Can you work these out from the model? Positions are in its coordinate system, mm. A direction names the side the tool comes from. Round coordinates to 2 decimals unless told otherwise and drop trailing zeros. Loops run counter-clockwise (first coordinate to the right, second up) from the corner with the lowest first, then second, coordinate; pieces in that order, holes last. Notation, with made-up numbers: M 28,1 L 35,1 A12 cw 35,11 Z; hole C 20.25,73 d9. An arc over 180 degrees is marked long. Use a Markdown table: item, result. Add a question column.
```python
from build123d import *

# Parameters (mm, degrees)
SKETCH2_W               = 1.4224
SKETCH2_H               = 1.27
CUT_EXTRUDE1_DEPTH      = 5.953
CUT_EXTRUDE1_DEPTH_BACK = 5.953


with BuildPart() as part:
    # Sketch1 → Revolve1 (revolve)
    with BuildSketch(Plane.XY):
        with BuildLine():
            Line((4.953, 22.1234), (2.032, 22.1234))
            Line((2.032, 22.1234), (2.032, 19.05))
            Line((2.032, 19.05), (2.4765, 19.05))
            Line((2.4765, 19.05), (2.4765, 0))
            Line((2.4765, 0), (4.953, 0))
            ThreePointArc((4.953, 0), (2.676809341, -1.50425402), (0, -2.032))
            Line((0, -2.032), (0, 24.1554))
            ThreePointArc((0, 24.1554), (2.676809341, 23.62765402), (4.953, 22.1234))
        make_face()
    revolve(axis=Axis((0, 24.1554, 0), (0, -1, 0)))

    # Sketch2 → Cut-Extrude1 (cut, two sides)
    with BuildSketch(Plane.XY) as cut_extrude1_sk:
        with Locations((0, 23.6474)):
            Rectangle(SKETCH2_W, SKETCH2_H)
    extrude(amount=CUT_EXTRUDE1_DEPTH, mode=Mode.SUBTRACT)
    extrude(cut_extrude1_sk.sketch, amount=-CUT_EXTRUDE1_DEPTH_BACK, mode=Mode.SUBTRACT)


solid = part.part
```
(1) I'm going to push flat-ended pins straight in: pin 1 (3 mm diameter, centred on x = -0.5, z = 1.5, fed in from -Y); pin 2 (2 mm diameter, centred on x = 2.5, z = -0.5, fed in from +Y); pin 3 (1 mm diameter, centred on y = 15.5, z = -2.5, fed in from +X); pin 4 (1 mm diameter, centred on x = -1, y = 3.5, fed in from -Z). Where does each tip first touch, or does it pass through?
(2) Thinking about a two-plate mould opening in X: for faces 1 (the face through (-0.44, 20.565, -1.984)), 2 (the face through (-2, 0, -2)), 3 (the face through (0.711, 23.4, -0.1)), which applies, released by +X, released by -X, zero draft, split by the parting line, or undercut?
(3) If I drill on probe 1 along Y at (x, z) = (1.5, -2.5); probe 2 along Y at (x, z) = (-3.5, 0.5); probe 3 along X at (y, z) = (23.25, 2), over which ranges is the centre line in solid material (lowest first)? Write a range as [from, to].
(4) Suppose I cut it at A-A on z = -2.75. List the corners of the cut face in (x, y) for me.
(5) Suppose I cut it at B-B on x = 0. List the corners of the cut face in (y, z) for me.
(6) On a 3-axis mill with a long thin cutter (end or side, diameter ignored), from which of +Z, -Z, +X, -X, +Y, -Y can I reach the whole of each face in a straight line? I mean faces 4 (the face through (0, 23.012, 0)), 5 (the face through (-0.322, 9.392, 2.455)). Say none if no direction works.
(7) Suppose I cut it at C-C on z = 0. List the corners of the cut face in (x, y) for me.
(8) Suppose I cut it at D-D on y = 19.75. List the corners of the cut face in (x, z) for me.
Results below:
| question | item | result |
|---|---|---|
| 1 | pin 1 | stops at y = -2.03 |
| 1 | pin 2 | stops at y = 23.98 |
| 1 | pin 3 | stops at x = 1.46 |
| 1 | pin 4 | stops at z = -2.43 |
| 2 | face 1 | split by the parting line |
| 2 | face 2 | zero draft |
| 2 | face 3 | undercut |
| 3 | probe 1 | y = [-1.4, 0], [22.12, 23.52] |
| 3 | probe 2 | y = [-1.08, 0], [22.12, 23.21] |
| 3 | probe 3 | x = [-2.82, -0.71], [0.71, 2.82] |
| 4 | outline | M -4.12,0 A6.49 ccw 4.12,0 Z; M -4.12,22.12 L 4.12,22.12 A6.49 ccw 0.71,23.56 L 0.71,23.01 L -0.71,23.01 L -0.71,23.56 A6.49 ccw Z |
| 5 | outline | M 0,-4.95 L 0,-2.48 L 19.05,-2.48 L 19.05,-2.03 L 22.12,-2.03 L 22.12,-4.95 A7.05 ccw 23.01,-3.85 L 23.01,3.85 A7.05 ccw 22.12,4.95 L 22.12,2.03 L 19.05,2.03 L 19.05,2.48 L 0,2.48 L 0,4.95 A7.05 ccw Z |
| 6 | face 4 | +Z, -Z, +Y |
| 6 | face 5 | none |
| 7 | outline | M -4.95,0 A7.05 ccw 4.95,0 L 2.48,0 L 2.48,19.05 L 2.03,19.05 L 2.03,22.12 L 4.95,22.12 A7.05 ccw 0.71,24.12 L 0.71,23.01 L -0.71,23.01 L -0.71,24.12 A7.05 ccw -4.95,22.12 L -2.03,22.12 L -2.03,19.05 L -2.48,19.05 L -2.48,0 Z |
| 8 | outline | C 0,0 d4.06 |
